```python
from build123d import *

# Parameters (mm, degrees)
PLACA_START                    = 46.75
SK_PLACA_W                     = 70
SK_PLACA_H                     = 160
PLACA_DEPTH                    = 6
EXTREMOS_START                 = 46.75
SK_EXTREMOS_R                  = 35
EXTREMOS_DEPTH                 = 6
PASANTES_M4_SEPARADORES_START  = 46.75
SK_PASANTES_M4_SEPARADORES_R   = 2.25
PASANTES_M4_SEPARADORES_DEPTH  = 6
ASIENTO_J3_START               = 38.75
SK_ASIENTO_J3_R                = 30
SK_ASIENTO_J3_R_2              = 17.5
ASIENTO_J3_DEPTH               = 8
PASO_ROTOR_J3_START            = 38.75
SK_PASO_ROTOR_J3_R             = 17.5
PASO_ROTOR_J3_DEPTH            = 14
PASANTES_M2_5_ESTATOR_J3_START = 38.75
SK_PASANTES_M2_5_ESTATOR_J3_R  = 1.45
PASANTES_M2_5_ESTATOR_J3_DEPTH = 14
CAJAS_M2_5_J3_START            = 50.25
SK_CAJAS_M2_5_J3_R             = 2.75
CAJAS_M2_5_J3_DEPTH            = 2.5
PASANTES_M4_SALIDA_J2_START    = 46.75
SK_PASANTES_M4_SALIDA_J2_R     = 2.25
PASANTES_M4_SALIDA_J2_DEPTH    = 6
CAJAS_M4_J2_START              = 49.25
SK_CAJAS_M4_J2_R               = 4
CAJAS_M4_J2_DEPTH              = 3.5
PASANTE_M3_CINCHO_START        = 46.75
SK_PASANTE_M3_CINCHO_R         = 1.7
PASANTE_M3_CINCHO_DEPTH        = 6


with BuildPart() as part:
    # Sk_Placa → Placa (new body)
    with BuildSketch(Plane(origin=(0, 0, 0), x_dir=(1, 0, 0), z_dir=(0, 1, 0)).offset(PLACA_START)):
        with Locations((0, -250)):
            Rectangle(SK_PLACA_W, SK_PLACA_H)
    extrude(amount=PLACA_DEPTH)

    # Sk_Extremos → Extremos (add)
    with BuildSketch(Plane(origin=(0, 0, 0), x_dir=(1, 0, 0), z_dir=(0, 1, 0)).offset(EXTREMOS_START)):
        with Locations((0, -170)):
            Circle(SK_EXTREMOS_R)
        with Locations((0, -330)):
            Circle(SK_EXTREMOS_R)
    extrude(amount=EXTREMOS_DEPTH)

    # Sk_Pasantes_M4_separadores → Pasantes_M4_separadores (cut)
    with BuildSketch(Plane(origin=(0, 0, 0), x_dir=(1, 0, 0), z_dir=(0, 1, 0)).offset(PASANTES_M4_SEPARADORES_START)):
        with Locations(Location((0, -250, 0), (0, 0, 270))):
            Circle(SK_PASANTES_M4_SEPARADORES_R)
        with Locations(Location((-22, -300, 0), (0, 0, 270))):
            Circle(SK_PASANTES_M4_SEPARADORES_R)
        with Locations(Location((22, -300, 0), (0, 0, 270))):
            Circle(SK_PASANTES_M4_SEPARADORES_R)
    extrude(amount=PASANTES_M4_SEPARADORES_DEPTH, mode=Mode.SUBTRACT)

    # Sk_Asiento_J3 → Asiento_J3 (add)
    with BuildSketch(Plane(origin=(0, 0, 0), x_dir=(1, 0, 0), z_dir=(0, 1, 0)).offset(ASIENTO_J3_START)):
        with Locations(Location((0, -330, 0), (0, 0, 270))):
            Circle(SK_ASIENTO_J3_R)
        with Locations(Location((0, -330, 0), (0, 0, 270))):
            Circle(SK_ASIENTO_J3_R_2, mode=Mode.SUBTRACT)
    extrude(amount=ASIENTO_J3_DEPTH)

    # Sk_Paso_rotor_J3 → Paso_rotor_J3 (cut)
    with BuildSketch(Plane(origin=(0, 0, 0), x_dir=(1, 0, 0), z_dir=(0, 1, 0)).offset(PASO_ROTOR_J3_START)):
        with Locations(Location((0, -330, 0), (0, 0, 270))):
            Circle(SK_PASO_ROTOR_J3_R)
    extrude(amount=PASO_ROTOR_J3_DEPTH, mode=Mode.SUBTRACT)

    # Sk_Pasantes_M2-5_estator_J3 → Pasantes_M2-5_estator_J3 (cut)
    with BuildSketch(Plane(origin=(0, 0, 0), x_dir=(1, 0, 0), z_dir=(0, 1, 0)).offset(PASANTES_M2_5_ESTATOR_J3_START)):
        with Locations(Location((20.289983175, -329.362361591, 0), (0, 0, 270))):
            Circle(SK_PASANTES_M2_5_ESTATOR_J3_R)
        with Locations(Location((14.798063137, -343.89630625, 0), (0, 0, 270))):
            Circle(SK_PASANTES_M2_5_ESTATOR_J3_R)
        with Locations(Location((0.637638409, -350.289983175, 0), (0, 0, 270))):
            Circle(SK_PASANTES_M2_5_ESTATOR_J3_R)
        with Locations(Location((-13.89630625, -344.798063137, 0), (0, 0, 270))):
            Circle(SK_PASANTES_M2_5_ESTATOR_J3_R)
        with Locations(Location((-20.289983175, -330.637638409, 0), (0, 0, 270))):
            Circle(SK_PASANTES_M2_5_ESTATOR_J3_R)
        with Locations(Location((-14.798063137, -316.10369375, 0), (0, 0, 270))):
            Circle(SK_PASANTES_M2_5_ESTATOR_J3_R)
        with Locations(Location((-0.637638409, -309.710016825, 0), (0, 0, 270))):
            Circle(SK_PASANTES_M2_5_ESTATOR_J3_R)
        with Locations(Location((13.89630625, -315.201936863, 0), (0, 0, 270))):
            Circle(SK_PASANTES_M2_5_ESTATOR_J3_R)
    extrude(amount=PASANTES_M2_5_ESTATOR_J3_DEPTH, mode=Mode.SUBTRACT)

    # Sk_Cajas_M2-5_J3 → Cajas_M2-5_J3 (cut)
    with BuildSketch(Plane(origin=(0, 0, 0), x_dir=(1, 0, 0), z_dir=(0, 1, 0)).offset(CAJAS_M2_5_J3_START)):
        with Locations(Location((20.289983175, -329.362361591, 0), (0, 0, 270))):
            Circle(SK_CAJAS_M2_5_J3_R)
        with Locations(Location((14.798063137, -343.89630625, 0), (0, 0, 270))):
            Circle(SK_CAJAS_M2_5_J3_R)
        with Locations(Location((0.637638409, -350.289983175, 0), (0, 0, 270))):
            Circle(SK_CAJAS_M2_5_J3_R)
        with Locations(Location((-13.89630625, -344.798063137, 0), (0, 0, 270))):
            Circle(SK_CAJAS_M2_5_J3_R)
        with Locations(Location((-20.289983175, -330.637638409, 0), (0, 0, 270))):
            Circle(SK_CAJAS_M2_5_J3_R)
        with Locations(Location((-14.798063137, -316.10369375, 0), (0, 0, 270))):
            Circle(SK_CAJAS_M2_5_J3_R)
        with Locations(Location((-0.637638409, -309.710016825, 0), (0, 0, 270))):
            Circle(SK_CAJAS_M2_5_J3_R)
        with Locations(Location((13.89630625, -315.201936863, 0), (0, 0, 270))):
            Circle(SK_CAJAS_M2_5_J3_R)
    extrude(amount=CAJAS_M2_5_J3_DEPTH, mode=Mode.SUBTRACT)

    # Sk_Pasantes_M4_salida_J2 → Pasantes_M4_salida_J2 (cut)
    with BuildSketch(Plane(origin=(0, 0, 0), x_dir=(1, 0, 0), z_dir=(0, 1, 0)).offset(PASANTES_M4_SALIDA_J2_START)):
        with Locations(Location((14.839084994, -167.808754572, 0), (0, 0, 270))):
            Circle(SK_PASANTES_M4_SALIDA_J2_R)
        with Locations(Location((9.317216704, -181.75540186, 0), (0, 0, 270))):
            Circle(SK_PASANTES_M4_SALIDA_J2_R)
        with Locations(Location((-5.52186829, -183.946647288, 0), (0, 0, 270))):
            Circle(SK_PASANTES_M4_SALIDA_J2_R)
        with Locations(Location((-14.839084994, -172.191245428, 0), (0, 0, 270))):
            Circle(SK_PASANTES_M4_SALIDA_J2_R)
        with Locations(Location((-9.317216704, -158.24459814, 0), (0, 0, 270))):
            Circle(SK_PASANTES_M4_SALIDA_J2_R)
        with Locations(Location((5.52186829, -156.053352712, 0), (0, 0, 270))):
            Circle(SK_PASANTES_M4_SALIDA_J2_R)
    extrude(amount=PASANTES_M4_SALIDA_J2_DEPTH, mode=Mode.SUBTRACT)

    # Sk_Cajas_M4_J2 → Cajas_M4_J2 (cut)
    with BuildSketch(Plane(origin=(0, 0, 0), x_dir=(1, 0, 0), z_dir=(0, 1, 0)).offset(CAJAS_M4_J2_START)):
        with Locations(Location((14.839084994, -167.808754572, 0), (0, 0, 270))):
            Circle(SK_CAJAS_M4_J2_R)
        with Locations(Location((9.317216704, -181.75540186, 0), (0, 0, 270))):
            Circle(SK_CAJAS_M4_J2_R)
        with Locations(Location((-5.52186829, -183.946647288, 0), (0, 0, 270))):
            Circle(SK_CAJAS_M4_J2_R)
        with Locations(Location((-14.839084994, -172.191245428, 0), (0, 0, 270))):
            Circle(SK_CAJAS_M4_J2_R)
        with Locations(Location((-9.317216704, -158.24459814, 0), (0, 0, 270))):
            Circle(SK_CAJAS_M4_J2_R)
        with Locations(Location((5.52186829, -156.053352712, 0), (0, 0, 270))):
            Circle(SK_CAJAS_M4_J2_R)
    extrude(amount=CAJAS_M4_J2_DEPTH, mode=Mode.SUBTRACT)

    # Sk_Pasante_M3_cincho → Pasante_M3_cincho (cut)
    with BuildSketch(Plane(origin=(0, 0, 0), x_dir=(1, 0, 0), z_dir=(0, 1, 0)).offset(PASANTE_M3_CINCHO_START)):
        with Locations(Location((-22, -230, 0), (0, 0, 270))):
            Circle(SK_PASANTE_M3_CINCHO_R)
    extrude(amount=PASANTE_M3_CINCHO_DEPTH, mode=Mode.SUBTRACT)


solid = part.part
```
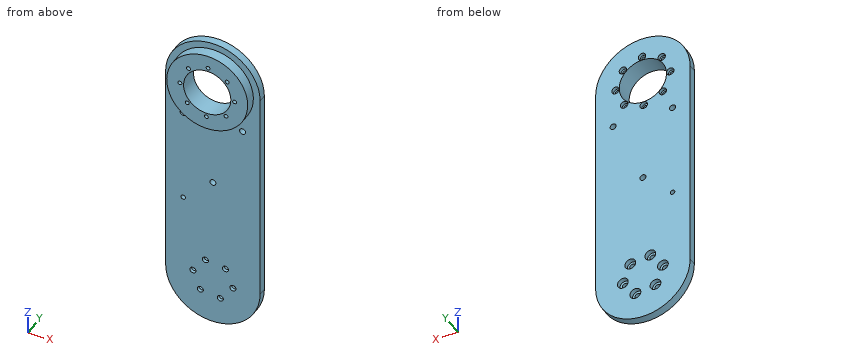
Work out the finished part from the listing and answer in its coordinate system (mm). Round coordinates to 2 decimals unless told otherwise and drop trailing zeros. Write each loop counter-clockwise with the first axis right and the second up, starting at its lowest first coordinate (ties: lowest second). Pieces come first, ordered by that corner, then holes. Notation, with made-up numbers: (14.25, 17) -> (57.25, 17) arc R25 cw to (57.25, 54) -> close; hole circle Ø7 at (39.25, -6.75). An arc over 180 degrees is marked (long way). Write each question's results on one line, items separated by ' | '.
1) Flat-ended cylindrical pins translate along their axes: pin 1 (9 mm diameter, centred on x = -9, z = 158, fed in from +Y); pin 2 (1 mm diameter, centred on x = -11, y = 43.5, fed in from -Z); pin 3 (4 mm diameter, centred on x = -16, z = 171, fed in from +Y); pin 4 (3 mm diameter, centred on x = 21.5, z = 329.5, fed in from +Y). Find the tip coordinate at first contact, or state that the pin passes through.
Findings:
pin 1: stops at y = 52.75 | pin 2: stops at z = 301.9 | pin 3: stops at y = 49.25 | pin 4: stops at y = 50.25
2) Consider line 1 along Z through (x, y) = (-13.5, 45); line 2 along X through (y, z) = (50.75, 343.5); line 3 along Y through (x, z) = (-31, 337). Determine where each line is inside the solid, lowest interval first. Write a range as [from, to].
Findings:
line 1: z = [303.21, 315.46], [316.75, 318.86], [341.14, 343.4], [346.19, 356.79] | line 2: x = [-32.29, -16.32], [-11.47, -11.14], [11.14, 12.08], [17.52, 32.29] | line 3: y = [46.75, 52.75]
3) The part is cut by section B-B (y = 44.25). State how many separate pieces and enclosed holes the cut face has, and give its area (3 significant figures).
Findings:
separate pieces: 1 | enclosed holes: 9 | area: 1,810 mm²
4) The part is cut by section A-A (z = 250). Write down the section's boundary in (x, y).
Findings:
outline: (-35, 46.75) -> (-2.25, 46.75) -> (-2.25, 52.75) -> (-35, 52.75) -> close; (2.25, 46.75) -> (35, 46.75) -> (35, 52.75) -> (2.25, 52.75) -> close
5) The part is cut by section C-C (z = 289.5). Write down the section's boundary in (x, y).
Findings:
outline: (-35, 46.75) -> (35, 46.75) -> (35, 52.75) -> (-35, 52.75) -> close
